Geometry: final body of the model. Coordinates: model frame, mm. Round coordinates to 2 decimals unless told otherwise and drop trailing zeros. Order: outer loops, then holes, each group sorted by start corner. A loop starts at its lowest first (then second) coordinate and runs counter-clockwise, first axis right, second up. Notation, with made-up numbers: M -24,-9.5 L 33,-9.5 A18 ccw 33,17.5 Z; hole C -37,89.25 d5. An arc over 180 degrees is marked long. Return JSON: item names as keys, results as strings. Group by question number.
Q1. Mould query, pull axis Y, two halves, no side actions, for faces 1 (the face through (20.03, -6.31, 0.99)), 2 (the face through (4.4, -4.4, 2)), 3 (the face through (-10.4, 9.88, 0.99)). Classes: released by +Y, released by -Y, zero draft, split by the parting line, or undercut.
Q2. Cut plane C-C on z = 1.1. Output: boundary loops of the cut face in (x, y).
Q3. Cut plane D-D on y = -13.5. Output: boundary loops of the cut face in (x, z).
Q4. Ray query, probe 1 along Y at (x, z) = (0, 1.25); probe 2 along Y at (x, z) = (12.5, 1.4); probe 3 along X at (y, z) = (-11.5, 0.6). Return the intervals inside material, ascending.
Q5. Cut plane A-A on y = 0. Output: boundary loops of the cut face in (x, z), and give its area (3 significant figures).
Q6. Contact query for flat-ended pins moving along their axis: pin 1 (1 mm diameter, centred on y = -14, z = 1.5, fed in from +X); pin 2 (15.5 mm diameter, centred on x = 0, y = 0, fed in from -Z); pin 3 (1 mm diameter, centred on x = 4.5, z = 0.5, fed in from +Y). Output: stop coordinate, or through.
Solid Edge part; units mm, degrees
sketch "Sketch1" plane through (0, 0, 0) normal (0, 0, 1) x (1, 0, 0)
  circle A0 centre (0, 0) radius 21
  circle A1 centre (0, 0) radius 6
  circle A2 centre (11.3137, 11.3137) radius 1.7
  circle A3 centre (-11.3137, 11.3137) radius 1.7
  circle A4 centre (-11.3137, -11.3137) radius 1.7
  circle A5 centre (11.3137, -11.3137) radius 1.7
extrude "Protrusion1" add sketch "Sketch1" along normal blind 2
Result sheet:
{
 "1": {"face 1": "split by the parting line", "face 2": "zero draft", "face 3": "undercut"},
 "2": {"outline": "C 0,0 d42; hole C -11.31,-11.31 d3.4; hole C -11.31,11.31 d3.4; hole C 0,0 d12; hole C 11.31,-11.31 d3.4; hole C 11.31,11.31 d3.4"},
 "3": {"outline": "M -16.09,0 L 16.09,0 L 16.09,2 L -16.09,2 Z"},
 "4": {"probe 1": "y = -21 to -6, 6 to 21", "probe 2": "y = -16.87 to -12.53, -10.1 to 10.1, 12.53 to 16.87", "probe 3": "x = -17.57 to -13, -9.62 to 9.62, 13 to 17.57"},
 "5": {"outline": "M -21,0 L -6,0 L -6,2 L -21,2 Z; M 6,0 L 21,0 L 21,2 L 6,2 Z", "area": "60.0 mm²"},
 "6": {"pin 1": "stops at x = 16.09", "pin 2": "stops at z = 0", "pin 3": "stops at y = 20.62"}
}
